The listing builds one solid part. Answer for the finished solid, in the listing's coordinates (mm). A direction names the side the tool comes from. Coordinates: 2 decimals unless noted, no trailing zeros. Order: outer loops, then holes, each group sorted by start corner. A loop starts at its lowest first (then second) coordinate and runs counter-clockwise, first axis right, second up. Notation, with made-up numbers: (83.5, 3) - (95.5, 3) arc R20 cw to (95.5, 42) - close; hole circle Ø10 at (-13, 27). An arc over 180 degrees is marked (long way). Use one line per item in the form item = value. Start each with the question number.
Item 1: Section B-B, the plane z = 2.55 is taken. Count the separate pieces of the cut face and the enclosed holes in it, and give its area (3 significant figures).
Item 2: Each of these flat-tipped pins is pushed along its axis until it touches: pin 1 Ø1 at (y, z) = (-75, 1.5) entering from -X; pin 2 Ø1 at (x, z) = (-168.5, 2) entering from +Y. Where does it stop, or does it pass through?
Item 3: Section C-C, the plane y = 34.5 is taken. Write down the section's boundary in (x, z) (3 decimals).
Item 4: Section A-A, the plane x = 104.5 is taken. Write down the section's boundary in (y, z) (3 decimals), and give its area (3 significant figures).
Item 5: A tool of negligible diameter and unlimited length cuts with its end or side. For faces 1 (the cylindrical face through (-142.46, -37.37, 1.61)), 2 (the flat face through (-52, 1, 3.175)), from which of +Z, -Z, +X, -X, +Y, -Y can it reach the whole face along a straight path? Write none if from no direction.
Item 6: Section D-D, the plane x = -42 is taken. Write down the section's boundary in (y, z) (3 decimals).
Item 7: The mould has two halves that part along X. Classify faces 3 (the cylindrical face through (32.532, 36.982, 1.61)), 4 (the flat face through (-52, 1, 0)): released by +X, released by -X, zero draft, split by the parting line, or undercut.
Item 8: Consider line 1 along X through (y, z) = (-7.5, 1.65); line 2 along Y through (x, z) = (-100.5, 0.3); line 3 along Y through (x, z) = (-26, 1). Determine where each line is inside the solid, lowest interval first. Write a range as [from, to].
from build123d import *

# Parameters (mm, degrees)
SKETCH1_W           = 89
SKETCH1_H           = 89
BOSS_EXTRUDE1_DEPTH = 3.175
FILLET1_R           = 25


with BuildPart() as part:
    # Sketch1 → Boss-Extrude1 (new body)
    with BuildSketch(Plane.XY):
        Polygon((-152.4, 69.85), (-177.8, 69.85), (-177.8, -69.85), (-152.4, -69.85), (-152.4, -88.9), (152.4, -88.9), (152.4, 88.9), (-152.4, 88.9), align=None)
        with Locations((96.05, 0)):
            Rectangle(SKETCH1_W, SKETCH1_H, mode=Mode.SUBTRACT)
        with Locations((-105.474, 0)):
            Rectangle(SKETCH1_W, SKETCH1_H, mode=Mode.SUBTRACT)
        with Locations((-4.839, 0)):
            Rectangle(SKETCH1_W, SKETCH1_H, mode=Mode.SUBTRACT)
    extrude(amount=BOSS_EXTRUDE1_DEPTH)

    # Fillet1
    fillet1_edges = [part.edges().sort_by_distance(p)[0] for p in [
        (140.55, -44.5, 1.5875),
        (140.55, 44.5, 1.5875),
        (51.55, 44.5, 1.5875),
        (51.55, -44.5, 1.5875),
        (-149.974, 44.5, 1.5875),
        (-149.974, -44.5, 1.5875),
        (-60.974, -44.5, 1.5875),
        (-60.974, 44.5, 1.5875),
        (-49.339, 44.5, 1.5875),
        (-49.339, -44.5, 1.5875),
        (39.661, -44.5, 1.5875),
        (39.661, 44.5, 1.5875),
    ]]
    fillet(fillet1_edges, radius=FILLET1_R)


solid = part.part
Response:
q1.separate_pieces = 1
q1.enclosed_holes = 3
q1.area = 35,600 mm2
q2.pin_1 = -152.4
q2.pin_2 = 69.85
q3.outline = (-177.8, 0) - (-144.974, 0) - (-144.974, 3.175) - (-177.8, 3.175) - close; (-65.974, 0) - (-44.339, 0) - (-44.339, 3.175) - (-65.974, 3.175) - close; (34.661, 0) - (56.55, 0) - (56.55, 3.175) - (34.661, 3.175) - close; (135.55, 0) - (152.4, 0) - (152.4, 3.175) - (135.55, 3.175) - close
q4.outline = (-88.9, 0) - (-44.5, 0) - (-44.5, 3.175) - (-88.9, 3.175) - close; (44.5, 0) - (88.9, 0) - (88.9, 3.175) - (44.5, 3.175) - close
q4.area = 282 mm2
q5.face_1 = +Z, -Z
q5.face_2 = +Z, +X, -X, +Y, -Y
q6.outline = (-88.9, 0) - (-37.194, 0) - (-37.194, 3.175) - (-88.9, 3.175) - close; (37.194, 0) - (88.9, 0) - (88.9, 3.175) - (37.194, 3.175) - close
q7.face_3 = undercut
q7.face_4 = zero draft
q8.line_1 = [-177.8, -149.97], [-60.97, -49.34], [39.66, 51.55], [140.55, 152.4]
q8.line_2 = [-88.9, -44.5], [44.5, 88.9]
q8.line_3 = [-88.9, -44.44], [44.44, 88.9]
